from build123d import *

# Parameters (mm, degrees)
F1_DEPTH = 31.75
F3_DEPTH = 25.4
F5_DEPTH = 12.7
F7_DEPTH = 12.7


with BuildPart() as f1:
    # F0 (on Top) → F1 (new body)
    with BuildSketch(Plane.XY):
        Polygon((0, 38.1), (0, 0), (31.75, 0), (31.75, 12.7), (69.85, 12.7), (69.85, 25.4), (31.75, 25.4), (31.75, 38.1), align=None)
    extrude(amount=F1_DEPTH)

    # F2 (on face) → F3 (cut)
    with BuildSketch(Plane.XZ.offset(-12.7)):
        Polygon((69.85, 31.75), (56.507498, 31.75), (69.85, 0), align=None)
    extrude(amount=-F3_DEPTH, mode=Mode.SUBTRACT)

    # F4 (on face) → F5 (cut)
    with BuildSketch(Plane.XZ):
        Polygon((31.75, 31.75), (19.05, 31.75), (31.75, 0), align=None)
    extrude(amount=-F5_DEPTH, mode=Mode.SUBTRACT)

    # F6 (on face) → F7 (cut)
    with BuildSketch(Plane(origin=(0, 38.1, 0), x_dir=(-1, 0, 0), z_dir=(0, 1, 0))):
        Polygon((-31.75, 31.75), (-31.75, 0), (-19.05, 31.75), align=None)
    extrude(amount=-F7_DEPTH, mode=Mode.SUBTRACT)


solid = f1.part
Here's how the part is built. I have some questions about the finished solid (model axes, mm). A direction names the side the tool comes from. Round coordinates to 2 decimals unless told otherwise and drop trailing zeros. Loops run counter-clockwise (first coordinate to the right, second up) from the corner with the lowest first, then second, coordinate; pieces in that order, holes last.
1. If we section it at D-D on x = 52: Write out the boundary of the cut face in (y, z).
Answer list:
outline: (12.7, 0) - (25.4, 0) - (25.4, 31.75) - (12.7, 31.75) - close
2. If we section it at A-A on x = 30: Write out the boundary of the cut face in (y, z) (3 decimals), plus the area to 3 significant figures.
Answer list:
outline: (0, 0) - (38.1, 0) - (38.1, 4.375) - (25.4, 4.375) - (25.4, 31.75) - (12.7, 31.75) - (12.7, 4.375) - (0, 4.375) - close
area: 514 mm2
3. Which directions (+Z, -Z, +X, -X, +Y, -Y) give clear straight access to the entire face, cutting with the end or side of a thin tool? Please do faces 1 (the face through (44, 12.7, 16)), 2 (the face through (45, 25.4, 16)), 3 (the face through (22, 19, 31.75)).
Answer list:
face 1: +Z, +X, -Y
face 2: +Z, +X, +Y
face 3: +Z, +X, -X, +Y, -Y
4. For P1, Ø9.5, axis at x = 46, z = 22.5, coming from the +Y side; P2, Ø6, axis at x = 61, y = 19, coming from the +Z side; P3, Ø4, axis at y = 17.5, z = 10.5, coming from the +X side, each with a flat end and sliding along its axis, tell me the tip position at first contact or that it passes through.
Answer list:
P1: stops at y = 25.4
P2: stops at z = 28.2
P3: stops at x = 66.28
5. If I drill on line 1 along Y through (x, z) = (56, 7.5); line 2 along X through (y, z) = (17, 3); line 3 along X through (y, z) = (30, 4.5), over which ranges is the centre line in solid material (lowest first)?
Answer list:
line 1: y = 12.7 to 25.4
line 2: x = 0 to 68.59
line 3: x = 0 to 29.95
6. If we section it at B-B on z = 8: Write out the boundary of the cut face in (x, y), plus the area to 3 significant figures.
Answer list:
outline: (0, 0) - (28.55, 0) - (28.55, 12.7) - (66.49, 12.7) - (66.49, 25.4) - (28.55, 25.4) - (28.55, 38.1) - (0, 38.1) - close
area: 1,570 mm2
7. If we section it at C-C on y = 21: Write out the boundary of the cut face in (x, z).
Answer list:
outline: (0, 0) - (69.85, 0) - (56.51, 31.75) - (0, 31.75) - close
